Could you check a few things on this model? Use its own coordinates, in mm. A direction names the side the tool comes from. Coordinates: 2 decimals unless noted, no trailing zeros. Order: outer loops, then holes, each group sorted by start corner. A loop starts at its lowest first (then second) coordinate and runs counter-clockwise, first axis right, second up. Notation, with made-up numbers: (36, 18) - (45, 18) arc R16 ccw to (45, 44) - close; hole circle Ø7 at (13.25, 0.5). An arc over 180 degrees is marked (long way). Answer as a JSON object with one key per item and string values. Group by question number.
(1) Please list where these lines run through material, in increasing order: probe 1 along Y at (x, z) = (-122.5, -65.5); probe 2 along Z at (x, y) = (146.5, -4).
(2) Will these pins go through, and if not, where does the flat tip stop? P1, Ø1.7, axis at y = -3.5, z = -7, coming from the -X side; P2, Ø3, axis at y = -4.5, z = -6.5, coming from the -X side; P3, Ø1.4, axis at y = -4.5, z = -5.5, coming from the -X side.
(3) Imagine slicing it at A-A, the plane z = 7. Write out the boundary of the cut face in (x, y), and give its area (3 significant figures).
(4) We'd pull the mould along Z, two halves only. Please class faces 1 (the cylindrical face through (48.074, -3.131, -24.946)), 2 (the flat face through (17, 0, -9)), 3 (the flat face through (112, -6.35, -15)): pulls with the +Z half, pulls with the -Z half, needs draft (parallel to the pull), parting line crosses it, or undercut.
(5) Which directions (+Z, -Z, +X, -X, +Y, -Y) give clear straight access to the entire face, cutting with the end or side of a thin tool? Please do faces 4 (the flat face through (201.5, -6.35, -0.6)), 5 (the cylindrical face through (172.537, -3.131, -9.608)).
from build123d import *

# Parameters (mm, degrees)
F4_DEPTH = 25.4
F1_R     = 12
F1_R_2   = 11.25
F1_R_3   = 10.5
F1_R_4   = 9.75
F1_R_5   = 9
F1_R_6   = 8.25
F1_R_7   = 7.5
F1_R_8   = 6.75
F1_R_9   = 6
F1_R_10  = 5.25
F5_DEPTH = 6.35
F2_R     = 14.2875
F2_R_2   = 11.90625
F2_R_3   = 10.715625
F2_R_4   = 9.525
F2_R_5   = 8.334375
F2_R_6   = 7.14375
F2_R_7   = 6.5484375
F2_R_8   = 5.953125
F2_R_9   = 4.7625
F6_DEPTH = 6.35


with BuildPart() as f4:
    # F3 (on Front) → F4 (new body)
    with BuildSketch(Plane.XZ):
        Polygon((238.1072341616, -69.85), (238.1072341616, 19.05), (-192.8318425985, 19.05), (-192.8318425985, -4.0414518917), (-192.8318425985, -69.85), align=None)
        with BuildLine():
            ThreePointArc((-182.3318425985, -4.0414518843), (-187.5818425948, -9.2914518843), (-192.8318425985, -4.0414518917))
            ThreePointArc((-192.8318425985, -4.0414518917), (-187.5818426022, 1.2085481157), (-182.3318425985, -4.0414518843))
        make_face(mode=Mode.SUBTRACT)
        with BuildLine():
            ThreePointArc((-182.3318425985, -4.0414518843), (-187.5818426022, 1.2085481157), (-192.8318425985, -4.0414518917))
            ThreePointArc((-192.8318425985, -4.0414518917), (-187.5818425948, -9.2914518843), (-182.3318425985, -4.0414518843))
        make_face()
    extrude(amount=-F4_DEPTH)

    # F1 (on Front) → F5 (join)
    with BuildSketch(Plane.XZ):
        with Locations((16.9928430942, -9.237604307)):
            Circle(F1_R)
        Polygon((16.9928430942, 0), (24.9928430942, -4.6188021535), (24.9928430942, -13.8564064606), (16.9928430942, -18.4752086141), (8.9928430942, -13.8564064606), (8.9928430942, -4.6188021535), align=None, mode=Mode.SUBTRACT)
        with Locations((-13.7432599701, -8.6602540378)):
            Circle(F1_R_2)
        Polygon((-13.7432599701, 0), (-6.2432599701, -4.3301270189), (-6.2432599701, -12.9903810568), (-13.7432599701, -17.3205080757), (-21.2432599701, -12.9903810568), (-21.2432599701, -4.3301270189), align=None, mode=Mode.SUBTRACT)
        with Locations((-42.4784353878, -8.0829037687)):
            Circle(F1_R_3)
        Polygon((-42.4784353878, 0), (-35.4784353878, -4.0414518843), (-35.4784353878, -12.124355653), (-42.4784353878, -16.1658075373), (-49.4784353878, -12.124355653), (-49.4784353878, -4.0414518843), align=None, mode=Mode.SUBTRACT)
        with Locations((-69.212550356, -7.5055534995)):
            Circle(F1_R_4)
        Polygon((-69.212550356, 0), (-62.712550356, -3.7527767497), (-62.712550356, -11.2583302492), (-69.212550356, -15.0111069989), (-75.712550356, -11.2583302492), (-75.712550356, -3.7527767497), align=None, mode=Mode.SUBTRACT)
        with Locations((-93.9454413277, -6.9282032303)):
            Circle(F1_R_5)
        Polygon((-93.9454413277, 0), (-87.9454413277, -3.4641016151), (-87.9454413277, -10.3923048454), (-93.9454413277, -13.8564064606), (-99.9454413277, -10.3923048454), (-99.9454413277, -3.4641016151), align=None, mode=Mode.SUBTRACT)
        with Locations((-116.6769037179, -6.3508529611)):
            Circle(F1_R_6)
        Polygon((-116.6769037179, 0), (-111.1769037179, -3.1754264805), (-111.1769037179, -9.5262794416), (-116.6769037179, -12.7017059222), (-122.1769037179, -9.5262794416), (-122.1769037179, -3.1754264805), align=None, mode=Mode.SUBTRACT)
        with Locations((-137.4066769023, -5.7735026919)):
            Circle(F1_R_7)
        Polygon((-137.4066769023, 0), (-132.4066769023, -2.8867513459), (-132.4066769023, -8.6602540378), (-137.4066769023, -11.5470053838), (-142.4066769023, -8.6602540378), (-142.4066769023, -2.8867513459), align=None, mode=Mode.SUBTRACT)
        with Locations((-156.1344216603, -5.1961524227)):
            Circle(F1_R_8)
        Polygon((-156.1344216603, 0), (-151.6344216603, -2.5980762114), (-151.6344216603, -7.7942286341), (-156.1344216603, -10.3923048454), (-160.6344216603, -7.7942286341), (-160.6344216603, -2.5980762114), align=None, mode=Mode.SUBTRACT)
        with Locations((-172.8596849761, -4.6188021535)):
            Circle(F1_R_9)
        Polygon((-172.8596849761, 0), (-168.8596849761, -2.3094010768), (-168.8596849761, -6.9282032303), (-172.8596849761, -9.237604307), (-176.8596849761, -6.9282032303), (-176.8596849761, -2.3094010768), align=None, mode=Mode.SUBTRACT)
        with Locations((-187.5818425985, -4.0414518843)):
            Circle(F1_R_10)
        Polygon((-187.5818425985, 0), (-184.0818425985, -2.0207259422), (-184.0818425985, -6.0621778265), (-187.5818425985, -8.0829037687), (-191.0818425985, -6.0621778265), (-191.0818425985, -2.0207259422), align=None, mode=Mode.SUBTRACT)
    extrude(amount=F5_DEPTH)

    # F2 (on Front) → F6 (join, through all)
    with BuildSketch(Plane.XZ):
        with Locations((51.1714122362, -10.9985226281)):
            Circle(F2_R)
        Polygon((51.1714122362, 0), (60.6964122362, -5.499261314), (60.6964122362, -16.4977839421), (51.1714122362, -21.9970452561), (41.6464122362, -16.4977839421), (41.6464122362, -5.499261314), align=None, mode=Mode.SUBTRACT)
        with Locations((85.1845816992, -9.1654355234)):
            Circle(F2_R_2)
        Polygon((85.1845816992, 0), (93.1220816992, -4.5827177617), (93.1220816992, -13.7481532851), (85.1845816992, -18.3308710468), (77.2470816992, -13.7481532851), (77.2470816992, -4.5827177617), align=None, mode=Mode.SUBTRACT)
        with Locations((114.9148765026, -8.248891971)):
            Circle(F2_R_3)
        Polygon((114.9148765026, 0), (122.0586265026, -4.1244459855), (122.0586265026, -12.3733379566), (114.9148765026, -16.4977839421), (107.7711265026, -12.3733379566), (107.7711265026, -4.1244459855), align=None, mode=Mode.SUBTRACT)
        with Locations((141.4662320164, -7.3323484187)):
            Circle(F2_R_4)
        Polygon((141.4662320164, 0), (147.8162320164, -3.6661742094), (147.8162320164, -10.9985226281), (141.4662320164, -14.6646968374), (135.1162320164, -10.9985226281), (135.1162320164, -3.6661742094), align=None, mode=Mode.SUBTRACT)
        with Locations((164.837657242, -6.4158048664)):
            Circle(F2_R_5)
        Polygon((164.837657242, 0), (170.393907242, -3.2079024332), (170.393907242, -9.6237072996), (164.837657242, -12.8316097328), (159.281407242, -9.6237072996), (159.281407242, -3.2079024332), align=None, mode=Mode.SUBTRACT)
        with Locations((185.0277321168, -5.499261314)):
            Circle(F2_R_6)
        Polygon((185.0277321168, 0), (189.7902321168, -2.749630657), (189.7902321168, -8.248891971), (185.0277321168, -10.9985226281), (180.2652321168, -8.248891971), (180.2652321168, -2.749630657), align=None, mode=Mode.SUBTRACT)
        with Locations((203.070830389, -5.0409895379)):
            Circle(F2_R_7)
        Polygon((203.070830389, 0), (207.436455389, -2.5204947689), (207.436455389, -7.5614843068), (203.070830389, -10.0819790757), (198.705205389, -7.5614843068), (198.705205389, -2.5204947689), align=None, mode=Mode.SUBTRACT)
        with Locations((219.5250878542, -4.5827177617)):
            Circle(F2_R_8)
        Polygon((219.5250878542, 0), (223.4938378542, -2.2913588808), (223.4938378542, -6.8740766425), (219.5250878542, -9.1654355234), (215.5563378542, -6.8740766425), (215.5563378542, -2.2913588808), align=None, mode=Mode.SUBTRACT)
        with Locations((233.3447341616, -3.6661742094)):
            Circle(F2_R_9)
        Polygon((233.3447341616, 0), (236.5197341616, -1.8330871047), (236.5197341616, -5.499261314), (233.3447341616, -7.3323484187), (230.1697341616, -5.499261314), (230.1697341616, -1.8330871047), align=None, mode=Mode.SUBTRACT)
    extrude(amount=F6_DEPTH)


solid = f4.part
Result set:
{
 "1": {"probe 1": "y = 0 to 25.4", "probe 2": "z = -15.42 to -11.76, -2.91 to 0.75"},
 "2": {"P1": "stops at x = -192.39", "P2": "stops at x = -192.74", "P3": "stops at x = -192.78"},
 "3": {"outline": "(-192.83, 0) - (238.11, 0) - (238.11, 25.4) - (-192.83, 25.4) - close", "area": "10,900 mm^2"},
 "4": {"face 1": "parting line crosses it", "face 2": "undercut", "face 3": "needs draft"},
 "5": {"face 4": "+Z, -Z, +X, -X, -Y", "face 5": "-Y"}
}
